For this review, take the finished solid that the model builds, in its own axes (mm). Face numbers are marked on the shaded views. A direction names the side the tool comes from. Coordinates: 2 decimals unless noted, no trailing zeros. Loops run counter-clockwise (first coordinate to the right, second up) from the corner with the lowest first, then second, coordinate; pieces in that order, holes last. Notation, with made-up numbers: M 56,79 L 113,79 A28 cw 113,109 Z; hole C 2.5,-19 d1. An arc over 180 degrees is marked long. Write each question's results on one line, items separated by ' | '. Start each with the question number.
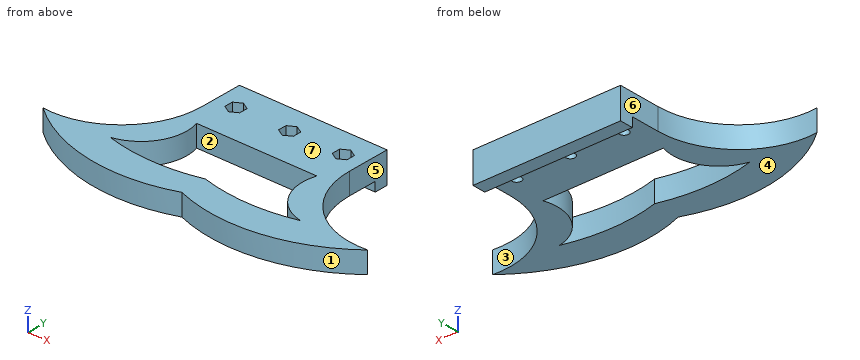
```python
from build123d import *

# Parameters (mm, degrees)
F0_W     = 55
F0_H     = 5
F0_H_2   = 11
F1_DEPTH = 8
F0_R     = 1.75
F2_DEPTH = 4
F3_DEPTH = 3.5


with BuildPart() as f1:
    # F0 (on Top) → F1 (new body)
    with BuildSketch(Plane.XY):
        with Locations((0, 5.5)):
            Rectangle(F0_W, F0_H)
        with Locations((0, -2.5)):
            Rectangle(F0_W, F0_H_2)
        Polygon((-20, 1.175426), (-17.25, -0.412287), (-17.25, -3.587713), (-20, -5.175426), (-22.75, -3.587713), (-22.75, -0.412287), align=None, mode=Mode.SUBTRACT)
        Polygon((0, -5.175426), (-2.75, -3.587713), (-2.75, -0.412287), (0, 1.175426), (2.75, -0.412287), (2.75, -3.587713), align=None, mode=Mode.SUBTRACT)
        Polygon((17.25, -3.587713), (17.25, -0.412287), (20, 1.175426), (22.75, -0.412287), (22.75, -3.587713), (20, -5.175426), align=None, mode=Mode.SUBTRACT)
        with BuildLine():
            Line((27.5, -8), (-27.5, -8))
            ThreePointArc((-27.5, -8), (-37.375388, -30.248595), (-60.5, -37.849623))
            ThreePointArc((-60.5, -37.849623), (-31.597894, -51.004383), (0, -47.849623))
            ThreePointArc((0, -47.849623), (31.597894, -51.004383), (60.5, -37.849623))
            ThreePointArc((60.5, -37.849623), (37.375388, -30.248595), (27.5, -8))
        make_face()
        with BuildLine():
            ThreePointArc((-35.5, -37.849623), (-24.035615, -29.871255), (-22.400142, -16))
            Line((-22.400142, -16), (22.400142, -16))
            ThreePointArc((22.400142, -16), (24.035615, -29.871255), (35.5, -37.849623))
            ThreePointArc((35.5, -37.849623), (17.75, -40.253807), (0, -37.849623))
            ThreePointArc((0, -37.849623), (-17.75, -40.253807), (-35.5, -37.849623))
        make_face(mode=Mode.SUBTRACT)
    extrude(amount=F1_DEPTH)

    # F0 (on Top) → F2 (join)
    with BuildSketch(Plane.XY):
        Polygon((-17.25, -3.587713), (-17.25, -0.412287), (-20, 1.175426), (-22.75, -0.412287), (-22.75, -3.587713), (-20, -5.175426), align=None)
        with Locations((-20, -2)):
            Circle(F0_R, mode=Mode.SUBTRACT)
        Polygon((-2.75, -0.412287), (-2.75, -3.587713), (0, -5.175426), (2.75, -3.587713), (2.75, -0.412287), (0, 1.175426), align=None)
        with Locations((0, -2)):
            Circle(F0_R, mode=Mode.SUBTRACT)
        Polygon((20, 1.175426), (17.25, -0.412287), (17.25, -3.587713), (20, -5.175426), (22.75, -3.587713), (22.75, -0.412287), align=None)
        with Locations((20, -2)):
            Circle(F0_R, mode=Mode.SUBTRACT)
    extrude(amount=F2_DEPTH)

    # F0 (on Top) → F3 (join)
    with BuildSketch(Plane.XY):
        with Locations((0, 5.5)):
            Rectangle(F0_W, F0_H)
    extrude(amount=-F3_DEPTH)


solid = f1.part
```
Q1. Take a section at B-B, the plane y = -2. Give the boundary of the cut face in (x, z).
Q2. For the marked faces 4, 5, 6 and 7, list the 3-axis set-ups (+Z, -Z, +X, -X, +Y, -Y) from which the entire face can be reached by the end or side of a thin tool; tool diameter is ignored.
Q3. The part is to be moulded in two halves that separate along Y. For the marked faces 1, 2 and 3, say which applies: pulls with the +Y half, pulls with the -Y half, needs draft (parallel to the pull), parting line crosses it, or undercut.
Q4. Take a section at D-D, the plane z = 2.5. Give the boundary of the cut face in (x, y).
Q5. Take a section at C-C, the plane y = -25.5. Give the boundary of the cut face in (x, z), then the cut area to 3 significant figures.
Q6. To check wall thickness, follow line 1 along Y through (x, z) = (-20, 1); line 2 along Y through (x, z) = (1, 6.5); line 3 along Z through (x, y) = (-18.5, -4.5). State the ranges of each line that lie inside material, in increasing order.
Q7. Take a section at A-A, the plane x = -30. Give the boundary of the cut face in (y, z), then the cut area to 3 significant figures.
Q8. Insertion check: P1, Ø5.5, axis at x = 20, y = -2, coming from the -Z side; P2, Ø1, axis at y = -1.5, z = 5.5, coming from the -X side; P3, Ø3, axis at x = -21, y = -3, coming from the +Z side; P4, Ø4, axis at x = 9.5, z = 4, coming from the -Y side. Each pin has a flat end and moves straight along its axis. Give the tip position at first contact, or say it passes through.
Results:
1) outline: M -27.5,0 L -21.75,0 L -21.75,4 L -22.75,4 L -22.75,8 L -27.5,8 Z; M -18.25,0 L -1.75,0 L -1.75,4 L -2.75,4 L -2.75,8 L -17.25,8 L -17.25,4 L -18.25,4 Z; M 1.75,0 L 18.25,0 L 18.25,4 L 17.25,4 L 17.25,8 L 2.75,8 L 2.75,4 L 1.75,4 Z; M 21.75,0 L 27.5,0 L 27.5,8 L 22.75,8 L 22.75,4 L 21.75,4 Z
2) face 4: -Z, +X, -X, -Y | face 5: +Z, -Z, +X, +Y | face 6: +Z, -Z, -X, +Y | face 7: +Z, +X, -X, +Y, -Y
3) face 1: pulls with the -Y half | face 2: undercut | face 3: pulls with the +Y half
4) outline: M -60.5,-37.85 A61 ccw 0,-47.85 A61 ccw 60.5,-37.85 A30 cw 27.5,-8 L 27.5,8 L -27.5,8 L -27.5,-8 A30 cw Z; hole M -35.5,-37.85 A66.73 ccw 0,-37.85 A66.73 ccw 35.5,-37.85 A17.02 cw 22.4,-16 L -22.4,-16 A17.02 cw Z; hole C -20,-2 d3.5; hole C 0,-2 d3.5; hole C 20,-2 d3.5
5) outline: M -33.13,0 L -22.19,0 L -22.19,8 L -33.13,8 Z; M 22.19,0 L 33.13,0 L 33.13,8 L 22.19,8 Z | area: 175 mm^2
6) line 1: -51.8 to -40.22, -16 to -3.75, -0.25 to 8 | line 2: -48.22 to -38.12, -16 to -4.6, 0.6 to 8 | line 3: 0 to 8
7) outline: M -51.25,0 L -39.12,0 L -39.12,8 L -51.25,8 Z; M -35.79,0 L -19.99,0 L -19.99,8 L -35.79,8 Z | area: 223 mm^2
8) P1: z = 0 | P2: x = -27.5 | P3: z = 8 | P4: y = -50.97
